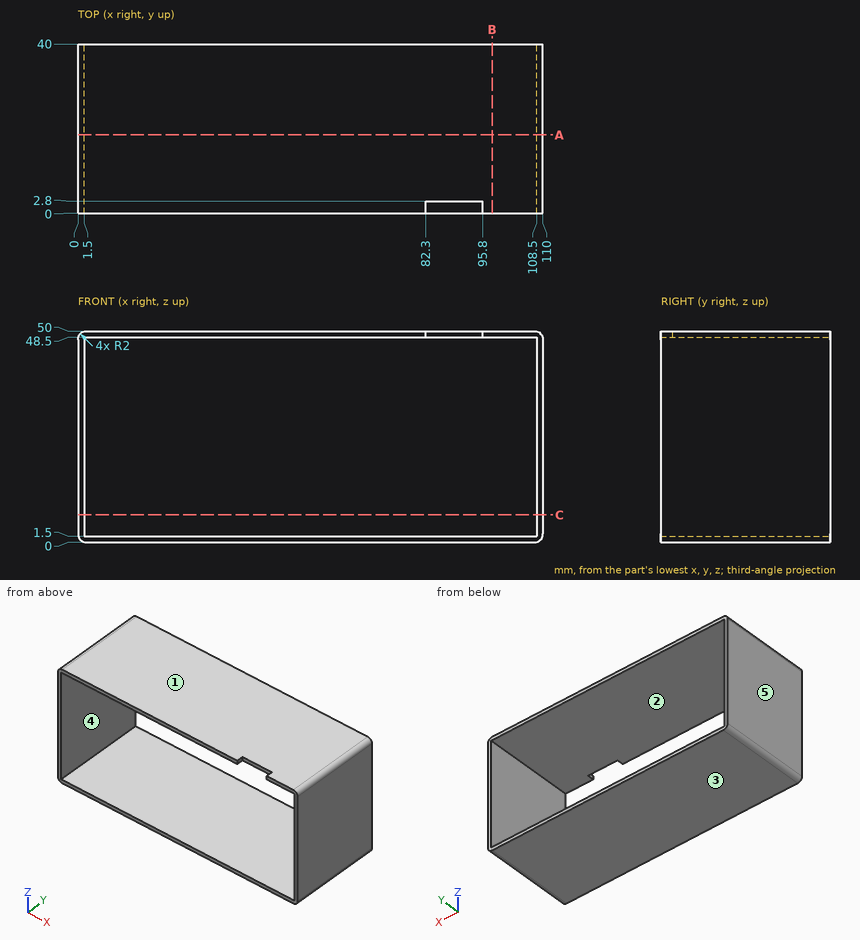
Here's the drawing with two shaded views (mm, measured from the low corner). I have some questions. A direction names the side the tool comes from. Give positions to 0.01 mm unless a question says otherwise; leave off trailing zeros. Order: outer loops, then holes, each group sorted by start corner. A loop starts at its lowest first (then second) coordinate and runs counter-clockwise, first axis right, second up.
Q1. For the marked faces 1 and 2, which set-ups out of +Z, -Z, +X, -X, +Y, -Y let a thin tool reach every point of the face, with its end or its side?
Q2. Suppose I cut it at A-A, the plane y = 18.5. Write out the boundary of the cut face in (x, z), and give its area (3 significant figures).
Q3. Suppose I cut it at B-B, the plane x = 98. Write out the boundary of the cut face in (y, z), and give its area (3 significant figures).
Q4. I'm going to push flat-ended pins straight in: P1, Ø1.6, axis at y = 2, z = 49.5, coming from the -X side; P2, Ø0.8, axis at x = 90.5, z = 49.5, coming from the -Y side. Where does each tip first touch, or does it pass through?
Q5. We'd pull the mould along X, two halves only. Please class the marked faces 3, 4 and 5: +X half, -X half, draft (parallel to the pull), parting line (faces both ways), or undercut.
Q6. If I drill on line 1 along Z through (x, y) = (27, 37.5); line 2 along X through (y, z) = (32, 28), over which ranges is the centre line in solid material (lowest first)?
Q7. Suppose I cut it at C-C, the plane z = 6.5. Write out the boundary of the cut face in (x, y).
Solution:
1. face 1: +Z, +X, -X, +Y, -Y
1. face 2: +Y, -Y
2. outline: (0, 2) arc R2 ccw to (2, 0) - (108, 0) arc R2 ccw to (110, 2) - (110, 48) arc R2 ccw to (108, 50) - (2, 50) arc R2 ccw to (0, 48) - close; hole (1.5, 1.5) - (108.5, 1.5) - (108.5, 48.5) - (1.5, 48.5) - close
2. area: 468 mm2
3. outline: (0, 0) - (40, 0) - (40, 1.5) - (0, 1.5) - close; (0, 48.5) - (40, 48.5) - (40, 50) - (0, 50) - close
3. area: 120 mm2
4. P1: stops at x = 0.13
4. P2: stops at y = 2.8
5. face 3: draft
5. face 4: undercut
5. face 5: -X half
6. line 1: z = 0 to 1.5, 48.5 to 50
6. line 2: x = 0 to 1.5, 108.5 to 110
7. outline: (0, 0) - (1.5, 0) - (1.5, 40) - (0, 40) - close; (108.5, 0) - (110, 0) - (110, 40) - (108.5, 40) - close
